```python
from build123d import *

# Parameters (mm, degrees)
EXTRUDE_12_DEPTH                  = 20
SKETCH_13_W                       = 54
SKETCH_13_H                       = 48
EXTRUDE_13_DEPTH                  = 22
EXTRUDE_START                     = -55
SKETCH_14_R                       = 30
EXTRUDE_14_DEPTH                  = 62
SKETCH_19_W                       = 50
SKETCH_19_H                       = 12
CUT_EXTRUDE_3_DEPTH               = 1
CUT_EXTRUDE_3_DEPTH_BACK          = 65
EXTRUDE_START_2                   = 6
SKETCH_20_R                       = 15
EXTRUDE_17_DEPTH                  = 78
SKETCH_21_R                       = 10
CUT_EXTRUDE_4_DEPTH               = 1.0000001
CUT_EXTRUDE_4_DEPTH_BACK          = 85
SKETCH_23_R                       = 17.5
CUT_EXTRUDE_7_DEPTH               = 48
SKETCH_25_R                       = 10
CUT_EXTRUDE_8_DEPTH               = 17
HOLE_WIZARD_13_0_13_2_D           = 13
HOLE_WIZARD_13_0_13_2_CSINK_D     = 13.05
HOLE_WIZARD_13_0_13_2_CSINK_ANGLE = 90


with BuildPart() as part:
    # Эскиз12 → Бобышка-Вытянуть12 (new body)
    with BuildSketch(Plane(origin=(0, 0, 0), x_dir=(1, 0, 0), z_dir=(0, 1, 0))):
        with BuildLine():
            Line((-49, -32), (49, -32))
            ThreePointArc((49, -32), (57.485281374, -28.485281374), (61, -20))
            Line((61, -20), (61, 20))
            ThreePointArc((61, 20), (57.485281374, 28.485281374), (49, 32))
            Line((49, 32), (-49, 32))
            ThreePointArc((-49, 32), (-57.485281374, 28.485281374), (-61, 20))
            Line((-61, 20), (-61, -20))
            ThreePointArc((-61, -20), (-57.485281374, -28.485281374), (-49, -32))
        make_face()
    extrude(amount=EXTRUDE_12_DEPTH)

    # Эскиз13 → Бобышка-Вытянуть13 (add)
    with BuildSketch(Plane(origin=(0, 20, 0), x_dir=(1, 0, 0), z_dir=(0, 1, 0))):
        Rectangle(SKETCH_13_W, SKETCH_13_H)
    extrude(amount=EXTRUDE_13_DEPTH)

    # Эскиз14 → Бобышка-Вытянуть14 (add)
    with BuildSketch(Plane.XY.offset(24).offset(EXTRUDE_START)):
        with Locations((0, 42)):
            Circle(SKETCH_14_R)
    extrude(amount=EXTRUDE_14_DEPTH)

    # Эскиз19 → Вырез-Вытянуть3 (cut, two sides)
    with BuildSketch(Plane.XY.offset(32)) as cut_extrude_3_sk:
        Rectangle(SKETCH_19_W, SKETCH_19_H)
    extrude(amount=CUT_EXTRUDE_3_DEPTH, mode=Mode.SUBTRACT)
    extrude(cut_extrude_3_sk.sketch, amount=-CUT_EXTRUDE_3_DEPTH_BACK, mode=Mode.SUBTRACT)

    # Эскиз20 → Бобышка-Вытянуть17 (add)
    with BuildSketch(Plane(origin=(0, 0, 0), x_dir=(1, 0, 0), z_dir=(0, 1, 0)).offset(EXTRUDE_START_2)):
        Circle(SKETCH_20_R)
    extrude(amount=EXTRUDE_17_DEPTH)

    # Эскиз21 → Вырез-Вытянуть4 (cut, two sides)
    with BuildSketch(Plane(origin=(0, 84, 0), x_dir=(1, 0, 0), z_dir=(0, 1, 0))) as cut_extrude_4_sk:
        Circle(SKETCH_21_R)
    extrude(amount=CUT_EXTRUDE_4_DEPTH, mode=Mode.SUBTRACT)
    extrude(cut_extrude_4_sk.sketch, amount=-CUT_EXTRUDE_4_DEPTH_BACK, mode=Mode.SUBTRACT)

    # Эскиз23 → Вырез-Вытянуть7 (cut)
    with BuildSketch(Plane.XY.offset(31)):
        with Locations((0, 42)):
            Circle(SKETCH_23_R)
    extrude(amount=-CUT_EXTRUDE_7_DEPTH, mode=Mode.SUBTRACT)

    # Эскиз25 → Вырез-Вытянуть8 (cut)
    with BuildSketch(Plane(origin=(0, 0, -31), x_dir=(-1, 0, 0), z_dir=(0, 0, -1))):
        with Locations((0, 42)):
            Circle(SKETCH_25_R)
    extrude(amount=-CUT_EXTRUDE_8_DEPTH, mode=Mode.SUBTRACT)

    # Диаметр отверстия Ø13.0 (13)2 (through all)
    with Locations(Plane(origin=(0, 20, 0), x_dir=(1, 0, 0), z_dir=(0, 1, 0))):
        with Locations((-47.963392627, 14), (-47.963392627, -16), (50.036607373, -16), (50.036607373, 14)):
            CounterSinkHole(HOLE_WIZARD_13_0_13_2_D / 2, HOLE_WIZARD_13_0_13_2_CSINK_D / 2, counter_sink_angle=HOLE_WIZARD_13_0_13_2_CSINK_ANGLE)


solid = part.part
```
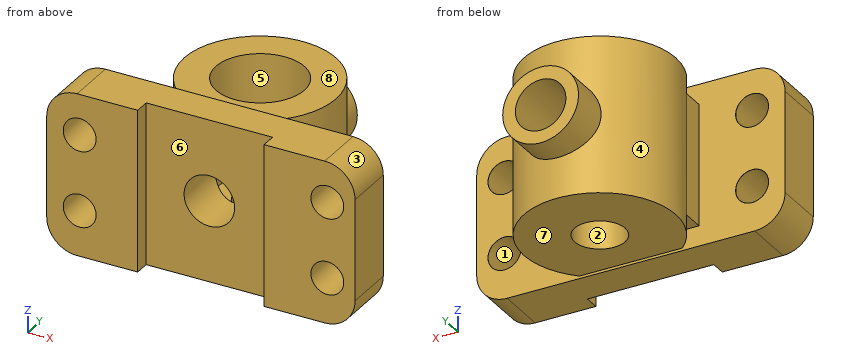
Work out the finished part from the listing and answer in its coordinate system (mm). Face numbers are marked on the shaded views. A direction names the side the tool comes from. Give positions to 0.01 mm unless a question says otherwise; leave off trailing zeros. Loops run counter-clockwise (first coordinate to the right, second up) from the corner with the lowest first, then second, coordinate; pieces in that order, holes last. Notation, with made-up numbers: M 58.5,30.25 L 87.5,30.25 A24 cw 87.5,40.25 Z; hole C 3,89.5 d11. An arc over 180 degrees is marked long. One line per item, written item: value. Start each with the question number.
1. Which of the six approach directions +Z, -Z, +X, -X, +Y, -Y give full straight-line access (tool end or side, diameter ignored) to the marked faces 4, 5, 6, 7 and 8?
2. Find section D-D (y = 10.5). Give the vertices of the cut face in (x, z).
3. Determine the mould class of the marked faces 1, 2 and 3 for opening direction Z: released by +Z, released by -Z, zero draft, split by the parting line, or undercut.
4. Each of these flat-tipped pins is pushed along its axis until it touches: P1, Ø7.5, axis at x = 25, y = 23, coming from the +Z side; P2, Ø21, axis at x = 50.04, z = 16, coming from the +Y side; P3, Ø3.5, axis at x = -22.5, y = 25.5, coming from the +Z side; P4, Ø10, axis at y = 50, z = 18, coming from the -X side. Where does it stop, or does it pass through?
5. Find section A-A (x = 0). Give the vertices of the cut face in (y, z), and give its area (3 significant figures).
6. Find section C-C (z = 0). Give the vertices of the cut face in (x, y), and give its area (3 significant figures).
7. Find the intervals of material crossed by probe 1 along X at (y, z) = (15.5, 16); probe 2 along X at (y, z) = (69.5, 0); probe 3 along Z at (x, y) = (-0.5, 68), in increasing order.
8. Find section B-B (y = 42). Give the vertices of the cut face in (x, z), and give its area (3 significant figures).
Reported:
1. face 4: none
1. face 5: +Z
1. face 6: +Z, -Z, -Y
1. face 7: -Z, +X, -X, +Y
1. face 8: +Z, +X, -X, +Y
2. outline: M -61,-20 A12 ccw -49,-32 L 49,-32 A12 ccw 61,-20 L 61,20 A12 ccw 49,32 L -49,32 A12 ccw -61,20 Z; hole C -47.96,-14 d13; hole C -47.96,16 d13; hole C 0,0 d20; hole C 50.04,-14 d13; hole C 50.04,16 d13
3. face 1: undercut
3. face 2: zero draft
3. face 3: released by +Z
4. P1: stops at z = 32
4. P2: stops at y = 20
4. P3: stops at z = 31
4. P4: stops at x = -29.85
5. outline: M 6,-32 L 20,-32 L 20,-31 L 32,-31 L 32,-17 L 24.5,-17 L 24.5,-10 L 6,-10 Z; M 6,10 L 24.5,10 L 24.5,31 L 20,31 L 20,32 L 6,32 Z; M 52,-31 L 72,-31 L 72,-15 L 84,-15 L 84,-10 L 59.5,-10 L 59.5,-17 L 52,-17 Z; M 59.5,10 L 84,10 L 84,15 L 72,15 L 72,31 L 59.5,31 Z
5. area: 1,660 mm²
6. outline: M -61,0 L -25,0 L -25,6 L -10,6 L -10,27.64 A17.5 cw -10,56.36 L -10,84 L -15,84 L -15,67.98 A30 ccw -27,28.92 L -27,20 L -61,20 Z; M 10,6 L 25,6 L 25,0 L 61,0 L 61,20 L 27,20 L 27,28.92 A30 ccw 15,67.98 L 15,84 L 10,84 L 10,56.36 A17.5 cw 10,27.64 Z
6. area: 3,330 mm²
7. probe 1: x = -61 to -54.46, -41.46 to 43.54, 56.54 to 61
7. probe 2: x = -15 to -10, 10 to 15
7. probe 3: z = -31 to -9.99, 9.99 to 31
8. outline: M -30,-31 L -10,-31 L -10,-17 L -17.5,-17 L -17.5,31 L -30,31 Z; M 10,-31 L 30,-31 L 30,31 L 17.5,31 L 17.5,-17 L 10,-17 Z
8. area: 1,760 mm²
